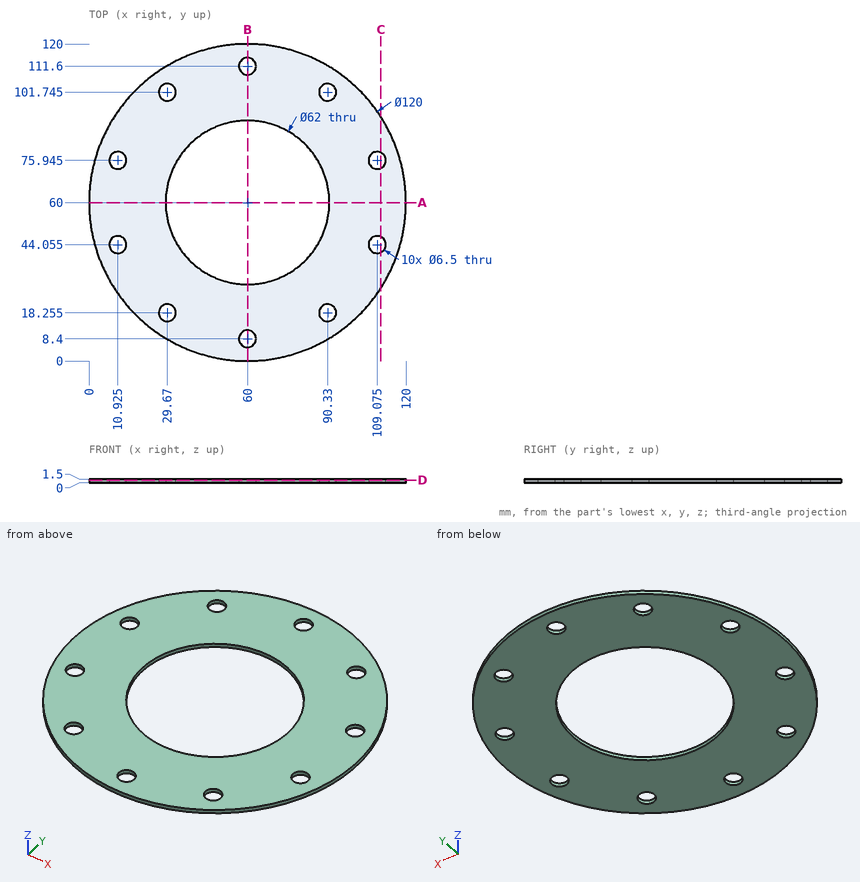
Geometry check sheet. Reference: drawing and pictorial views, mm from the part's lowest x, y, z. Give positions to 0.01 mm unless a question says otherwise; leave off trailing zeros. Order: outer loops, then holes, each group sorted by start corner. A loop starts at its lowest first (then second) coordinate and runs counter-clockwise, first axis right, second up. Notation, with made-up numbers: (54.5, -5.5) -> (63.5, -5.5) arc R22 ccw to (63.5, 16.5) -> close; hole circle Ø7 at (63.25, 3). An arc over 180 degrees is marked (long way). Use CSV: the item, a comma, the result in double quotes. Start each with the question number.
1) Sectioned sample at A-A, the plane y = 60. Record the boundary of the cut face in (x, z).
2) Sectioned sample at D-D, the plane z = 1.05. Give the number of separate pieces and of enclosed holes in the cut face, plus the area to 3 significant figures.
3) Sectioned sample at B-B, the plane x = 60. Record the boundary of the cut face in (y, z).
4) Material ranges on line 1 (Y direction, x = 60, z = 0.7); line 2 (Y direction, x = 12, z = 0.5) (1 decimal); line 3 (X direction, y = 101, z = 0.6) (1 decimal), recorded low to high. Write a range as from..to.
5) Sectioned sample at C-C, the plane x = 110.5. Record the boundary of the cut face in (y, z) (1 decimal).
Recorded:
1,outline,"(0, 0) -> (29, 0) -> (29, 1.5) -> (0, 1.5) -> close; (91, 0) -> (120, 0) -> (120, 1.5) -> (91, 1.5) -> close"
2,separate pieces,"1"
2,enclosed holes,"11"
2,area,"7,960 mm2"
3,outline,"(0, 0) -> (5.15, 0) -> (5.15, 1.5) -> (0, 1.5) -> close; (11.65, 0) -> (29, 0) -> (29, 1.5) -> (11.65, 1.5) -> close; (91, 0) -> (108.35, 0) -> (108.35, 1.5) -> (91, 1.5) -> close; (114.85, 0) -> (120, 0) -> (120, 1.5) -> (114.85, 1.5) -> close"
4,line 1,"0..5.15, 11.65..29, 91..108.35, 114.85..120"
4,line 2,"24..41, 47.1..72.9, 79..96"
4,line 3,"16.2..26.5, 32.8..87.2, 93.5..103.8"
5,outline,"(27.6, 0) -> (41.1, 0) -> (41.1, 1.5) -> (27.6, 1.5) -> close; (47, 0) -> (73, 0) -> (73, 1.5) -> (47, 1.5) -> close; (78.9, 0) -> (92.4, 0) -> (92.4, 1.5) -> (78.9, 1.5) -> close"
